from build123d import *

# Parameters (mm, degrees)
F0_R     = 11.1125
F1_DEPTH = 19.304
F3_DEPTH = 19.304


with BuildPart() as f1:
    # F0 (on Front) → F1 (new body)
    with BuildSketch(Plane.XZ):
        with BuildLine():
            Line((-66.04, 0), (0, 0))
            Line((0, 0), (0, 53.34))
            ThreePointArc((0, 53.34), (-33.02, 86.36), (-66.04, 53.34))
            Line((-66.04, 53.34), (-66.04, 0))
        make_face()
        with Locations((-33.02, 53.34)):
            Circle(F0_R, mode=Mode.SUBTRACT)
    extrude(amount=F1_DEPTH)

    # F2 (on Top) → F3 (join)
    with BuildSketch(Plane.XY):
        Polygon((0, -38.608), (0, 0), (-66.04, 0), (-66.04, -38.608), (-47.244, -38.608), (-47.244, -28.956), (-18.796, -28.956), (-18.796, -38.608), align=None)
    extrude(amount=F3_DEPTH)


solid = f1.part
Could you check a few things on this model? Use its own coordinates, in mm. A direction names the side the tool comes from. Coordinates: 2 decimals unless noted, no trailing zeros. Order: outer loops, then holes, each group sorted by start corner. A loop starts at its lowest first (then second) coordinate and runs counter-clockwise, first axis right, second up. Notation, with made-up numbers: (42, -11) -> (46, -11) arc R18 cw to (46, 4) -> close; hole circle Ø10 at (-11, 10). An arc over 180 degrees is marked (long way). One line per question, with ' | ' between items.
Q1. I'm going to push flat-ended pins straight in: P1, Ø1.5, axis at x = -49, y = -5.5, coming from the +Z side; P2, Ø6, axis at y = -28.5, z = 25, coming from the +X side; P3, Ø9.5, axis at x = -27.5, y = -32, coming from the +Z side; P4, Ø15.5, axis at x = -34, z = 10, coming from the -Y side. Where does each tip first touch, or does it pass through?
Return value:
P1: z = 82.64 | P2: through | P3: z = 19.3 | P4: y = -28.96
Q2. Imagine slicing it at D-D on y = -3. Please give me the cut outline in (x, z) (1 decimal).
Return value:
outline: (-66, 0) -> (0, 0) -> (0, 53.3) arc R33 ccw to (-66, 53.3) -> close; hole circle Ø22.2 at (-33, 53.3)
Q3. Thinking about a two-plate mould opening in X: for faces 4 (the face through (-33, -19.304, 38)), 5 (the face through (-47.244, -34, 10)), 6 (the face through (0, -15, 20)), which applies, pulls with the +X half, pulls with the -X half, needs draft (parallel to the pull), parting line crosses it, or undercut?
Return value:
face 4: needs draft | face 5: undercut | face 6: pulls with the +X half
Q4. Imagine slicing it at B-B on x = -33.02. Please give me the cut outline in (y, z).
Return value:
outline: (-28.96, 0) -> (0, 0) -> (0, 42.23) -> (-19.3, 42.23) -> (-19.3, 19.3) -> (-28.96, 19.3) -> close; (-19.3, 64.45) -> (0, 64.45) -> (0, 86.36) -> (-19.3, 86.36) -> close
Q5. Imagine slicing it at A-A on y = -32.5. Please give me the cut outline in (x, z), and give its area (3 significant figures).
Return value:
outline: (-66.04, 0) -> (-47.24, 0) -> (-47.24, 19.3) -> (-66.04, 19.3) -> close; (-18.8, 0) -> (0, 0) -> (0, 19.3) -> (-18.8, 19.3) -> close | area: 726 mm²
Q6. If I drill on L1, parallel to Z at x = -33.02, y = -10.75; L2, parallel to X at y = -36.5, z = 18; L3, parallel to X at y = -9, z = 53, over which ranges is the centre line in solid material (lowest first)?
Return value:
L1: 0 to 42.23, 64.45 to 86.36 | L2: -66.04 to -47.24, -18.8 to 0 | L3: -66.04 to -44.13, -21.91 to 0
Q7. Imagine slicing it at C-C on z = 8.5. Please give me the cut outline in (x, y).
Return value:
outline: (-66.04, -38.61) -> (-47.24, -38.61) -> (-47.24, -28.96) -> (-18.8, -28.96) -> (-18.8, -38.61) -> (0, -38.61) -> (0, 0) -> (-66.04, 0) -> close
Q8. On a 3-axis mill with a long thin cutter (end or side, diameter ignored), from which of +Z, -Z, +X, -X, +Y, -Y can I reach the whole of each face in a straight line? I mean faces 1 (the face through (-33, -28.956, 10)), 2 (the face through (-33, -27, 19.304)), 3 (the face through (-22.755, -9.517, 49.084)). Say none if no direction works.
Return value:
face 1: +Z, -Z, -Y | face 2: +Z, +X, -X, -Y | face 3: +Y, -Y
